Source: CAD feature listing. Evaluate the final solid. Frame: model axes, mm. Face numbers are marked on the shaded views. Coordinates: 2 decimals unless noted, no trailing zeros. Loops run counter-clockwise (first coordinate to the right, second up) from the corner with the lowest first, then second, coordinate; pieces in that order, holes last.
Item 1: Section query C-C, the plane x = -4. Return the cut outline in (y, z) (3 decimals).
Item 2: Section query A-A, the plane x = 0. Return the cut outline in (y, z) (3 decimals).
Item 3: Pin query (flat end, axial travel): pin 1 Ø1.5 at (x, z) = (0.5, 2.5) entering from -Y. Return the tip coordinate at first contact, or that it passes through.
Item 4: Line query: probe 1 along Y at (x, z) = (0, 1.45); probe 2 along X at (y, z) = (-1.5, 0.3); probe 3 along X at (y, z) = (2.25, 3). Output: solid intervals per line, ascending.
Item 5: Pull-direction query (Y, two-part tool) for the marked faces 1, 2, 3 and 4; classes: +Y half, -Y half, draft (parallel to the pull), parting line (faces both ways), or undercut.
Item 6: Section query D-D, the plane z = 1.35. Return the cut outline in (x, y) (1 decimal).
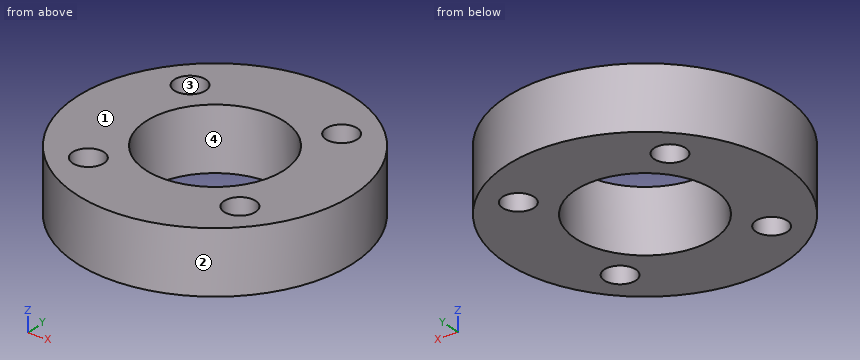
Autodesk Inventor part; units mm, degrees
ref_plane "YZ Plane" through (0, 0, 0) normal (1, 0, 0) x (0, 1, 0)
ref_plane "XZ Plane" through (0, 0, 0) normal (0, 1, 0) x (-1, 0, 0)
ref_plane "XY Plane" through (0, 0, 0) normal (0, 0, 1) x (1, 0, 0)
sketch "Sketch1" plane through (0, 0, 0) normal (0, 0, 1) x (1, 0, 0)
  circle A0 centre (0, 0) radius 3.5
  circle A1 centre (0, 0) radius 7
  circle A2 centre (3.9313, -3.4792) radius 0.7937
  circle A3 centre (3.4792, 3.9313) radius 0.7937
  circle A4 centre (-3.9313, 3.4792) radius 0.7937
  circle A5 centre (-3.4792, -3.9313) radius 0.7937
  dimension "d0" = 7
  dimension "d1" = 14
  dimension "d2" = 1.5875
  dimension "d3" = 0.956
  dimension "d6" = 360
  dimension "d10" = 0.956
  dimension "d11" = 0.956
  dimension "d12" = 0.956
  dimension "d13" = 5.8368
  dimension "d14" = 5.8368
  dimension "d15" = 5.8368
extrude "Extrusion1" add sketch "Sketch1" along normal blind 3.175
properties part number "gear ring"
Verdict:
1. outline: (-5.745, 0) - (-4.53, 0) - (-4.53, 3.175) - (-5.745, 3.175) - close; (-3.332, 0) - (2.688, 0) - (2.688, 3.175) - (-3.332, 3.175) - close; (4.27, 0) - (5.745, 0) - (5.745, 3.175) - (4.27, 3.175) - close
2. outline: (-7, 0) - (-3.5, 0) - (-3.5, 3.175) - (-7, 3.175) - close; (3.5, 0) - (7, 0) - (7, 3.175) - (3.5, 3.175) - close
3. pin 1: stops at y = -7
4. probe 1: y = -7 to -3.5, 3.5 to 7
4. probe 2: x = -6.84 to -3.16, 3.16 to 6.84
4. probe 3: x = -6.63 to -2.68, 2.68 to 6.63
5. face 1: draft
5. face 2: parting line
5. face 3: undercut
5. face 4: undercut
6. outline: circle Ø14 at (0, 0); hole circle Ø1.6 at (-3.9, 3.5); hole circle Ø1.6 at (-3.5, -3.9); hole circle Ø7 at (0, 0); hole circle Ø1.6 at (3.5, 3.9); hole circle Ø1.6 at (3.9, -3.5)
